from build123d import *

# Parameters (mm, degrees)
F0_W     = 850.9
F0_H     = 736.6
F1_DEPTH = 19.05
F2_W     = 6.35
F2_H     = 12.7
F4_DEPTH = 736.601
F3_W     = 12.7
F3_H     = 6.35
F5_DEPTH = 850.901


with BuildPart() as f1:
    # F0 (on Front) → F1 (new body)
    with BuildSketch(Plane.XZ):
        with Locations((425.45, 368.3)):
            Rectangle(F0_W, F0_H)
    extrude(amount=F1_DEPTH)

    # F2 (on face) → F4 (cut, through all)
    with BuildSketch(Plane(origin=(0, 0, 0), x_dir=(1, 0, 0), z_dir=(0, 0, -1))):
        with Locations((847.725, 12.7)):
            Rectangle(F2_W, F2_H)
        with Locations((3.175, 12.7)):
            Rectangle(F2_W, F2_H)
    extrude(amount=-F4_DEPTH, mode=Mode.SUBTRACT)

    # F3 (on face) → F5 (cut, through all)
    with BuildSketch(Plane.YZ.offset(850.9)):
        with Locations((-12.7, 733.425)):
            Rectangle(F3_W, F3_H)
    extrude(amount=-F5_DEPTH, mode=Mode.SUBTRACT)


solid = f1.part
Could you check a few things on this model? Use its own coordinates, in mm. Give positions to 0.01 mm unless a question says otherwise; leave off trailing zeros. Loops run counter-clockwise (first coordinate to the right, second up) from the corner with the lowest first, then second, coordinate; pieces in that order, holes last. Notation, with made-up numbers: M -1,32.5 L 39,32.5 A14 ccw 39,50.5 Z; hole C 5.25,14.25 d4. An arc over 180 degrees is marked long. Answer as a JSON object with one key per item and string values.
Q1. For P1, Ø1, axis at y = -7.5, z = 100.5, coming from the +X side; P2, Ø10, axis at x = 321, y = -15, coming from the +Z side; P3, Ø3, axis at y = -8.5, z = 652, coming from the -X side, each with a flat end and sliding along its axis, tell me the tip position at first contact or that it passes through.
Values found:
{"P1": "stops at x = 844.55", "P2": "stops at z = 730.25", "P3": "stops at x = 6.35"}
Q2. If I drill on probe 1 along X at (y, z) = (-6.75, 688); probe 2 along Z at (x, y) = (223.5, -14.5), over which ranges is the centre line in solid material (lowest first)? Write a range as [from, to].
Values found:
{"probe 1": "x = [6.35, 844.55]", "probe 2": "z = [0, 730.25]"}
Q3. Suppose I cut it at A-A, the plane y = -11.25. List the corners of the cut face in (x, z) for me.
Values found:
{"outline": "M 6.35,0 L 844.55,0 L 844.55,730.25 L 6.35,730.25 Z"}
